from build123d import *

# Parameters (mm, degrees)
BOSS_EXTRUDE1_DEPTH     = 9.525
CUT_EXTRUDE1_DEPTH      = 10.525
CUT_EXTRUDE1_DEPTH_BACK = 10.525


with BuildPart() as part:
    # Sketch1 → Boss-Extrude1 (new body, symmetric)
    with BuildSketch(Plane.XY):
        Polygon((0, 0), (-41.275, 0), (0, 31.75), align=None)
    extrude(amount=BOSS_EXTRUDE1_DEPTH, both=True)

    # Sketch2 → Cut-Extrude1 (cut, two sides)
    with BuildSketch(Plane.XY) as cut_extrude1_sk:
        Polygon((-3.175, 5.177841223), (-16.255709614, 15.239925542), (-3.175, 25.302009861), align=None)
        Polygon((-5.77869359, 3.175), (-18.859403205, 13.237084319), (-31.940112819, 3.175), align=None)
    extrude(amount=CUT_EXTRUDE1_DEPTH, mode=Mode.SUBTRACT)
    extrude(cut_extrude1_sk.sketch, amount=-CUT_EXTRUDE1_DEPTH_BACK, mode=Mode.SUBTRACT)


solid = part.part
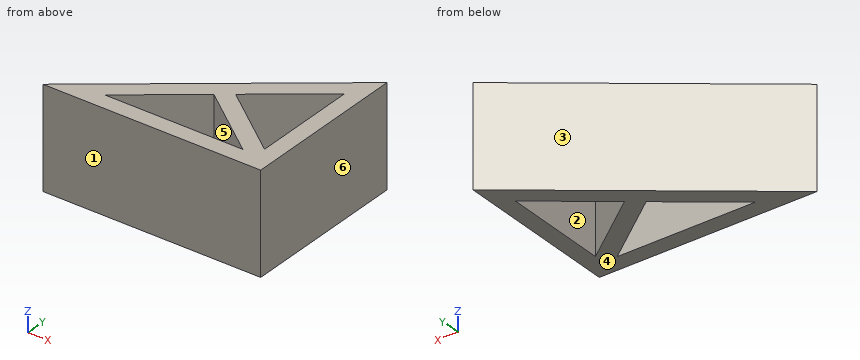
Geometry: final body of the model. Coordinates: model frame, mm. Face numbers are marked on the shaded views. A direction names the side the tool comes from. Round coordinates to 2 decimals unless told otherwise and drop trailing zeros. Loops run counter-clockwise (first coordinate to the right, second up) from the corner with the lowest first, then second, coordinate; pieces in that order, holes last. Notation, with made-up numbers: (6.5, 21) - (19.5, 21) arc R9 ccw to (19.5, 33) - close; hole circle Ø7 at (-27.5, 38). An arc over 180 degrees is marked (long way). Write each question's results on one line, items separated by ' | '. Start each with the question number.
1) Cut plane C-C on x = -15. Return loops of the section in (y, z) (3 decimals), then the cut area to 3 significant figures.
2) Line query: probe 1 along Y at (x, z) = (-9.5, -3.25) (3 decimals); probe 2 along Y at (x, z) = (-8.5, 7.5) (3 decimals); probe 3 along X at (y, z) = (11, -1.75) (3 decimals). Output: solid intervals per line, ascending. Write a range as [from, to].
3) Cut plane A-A on z = 4.75. Return loops of the section in (x, y) (3 decimals), then the cut area to 3 significant figures.
4) Mould query, pull axis X, two halves, no side actions, for the marked faces 3, 4, 5 and 6. Classes: released by +X, released by -X, zero draft, split by the parting line, or undercut.
5) Cut plane D-D on y = 21. Return loops of the section in (x, z) (3 decimals).
6) Cut plane B-B on y = 10.5. Return loops of the section in (x, z) (3 decimals).
7) First-contact query: P1, Ø8, axis at y = 9.5, z = 0, coming from the -X side (3 decimals); P2, Ø3, axis at x = -28, z = -7, coming from the -Y side; P3, Ø1.5, axis at y = 27, z = -3, coming from the -X side. Flat tips, straight axial feed; report the tip coordinate or a pass-through.
8) Access query for the marked faces 1 and 2. Directions: +Z, -Z, +X, -X, +Y, -Y. A direction counts if a zero-diameter tool reaches every point of the face in a straight line with its end or side. Return the directions, or none.
Verdict:
1) outline: (0, -9.525) - (3.175, -9.525) - (3.175, 9.525) - (0, 9.525) - close; (10.268, -9.525) - (14.274, -9.525) - (14.274, 9.525) - (10.268, 9.525) - close; (16.206, -9.525) - (20.212, -9.525) - (20.212, 9.525) - (16.206, 9.525) - close | area: 213 mm2
2) probe 1: y = [0, 3.175], [6.038, 10.043], [20.437, 24.442] | probe 2: y = [0, 3.175], [5.268, 9.274], [21.206, 25.212] | probe 3: x = [-26.975, -21.768], [-15.951, -10.744], [-3.175, 0]
3) outline: (-41.275, 0) - (0, 0) - (0, 31.75) - close; hole (-31.94, 3.175) - (-5.779, 3.175) - (-18.859, 13.237) - close; hole (-16.256, 15.24) - (-3.175, 5.178) - (-3.175, 25.302) - close | area: 392 mm2
4) face 3: released by -X | face 4: zero draft | face 5: undercut | face 6: released by +X
5) outline: (-13.975, -9.525) - (-8.768, -9.525) - (-8.768, 9.525) - (-13.975, 9.525) - close; (-3.175, -9.525) - (0, -9.525) - (0, 9.525) - (-3.175, 9.525) - close
6) outline: (-27.625, -9.525) - (-22.418, -9.525) - (-22.418, 9.525) - (-27.625, 9.525) - close; (-15.301, -9.525) - (-10.094, -9.525) - (-10.094, 9.525) - (-15.301, 9.525) - close; (-3.175, -9.525) - (0, -9.525) - (0, 9.525) - (-3.175, 9.525) - close
7) P1: stops at x = -34.125 | P2: stops at y = 0 | P3: stops at x = -7.15
8) face 1: +Z, -Z, +X, -X, -Y | face 2: +Z, -Z
